```python
from build123d import *

# Parameters (mm, degrees)
SKETCH_1_R      = 1.5
SKETCH_1_R_2    = 7.9
SKETCH_1_R_3    = 1.25
SKETCH_1_W      = 6
SKETCH_1_H      = 10
SKETCH_1_W_2    = 10
SKETCH_1_H_2    = 6
EXTRUDE_1_DEPTH = 6


with BuildPart() as part:
    # Эскиз1 → Бобышка-Вытянуть1 (new body)
    with BuildSketch(Plane.XY):
        with BuildLine():
            Line((146.861398458, 191.532325026), (172.897783364, 191.532325026))
            ThreePointArc((172.897783364, 191.532325026), (177.076317747, 189.745999648), (178.804179186, 185.542952802))
            Line((178.804179186, 185.542952802), (178.804179186, -196.675834418))
            ThreePointArc((178.804179186, -196.675834418), (176.892140189, -200.429470569), (172.897783364, -201.767674974))
            Line((172.897783364, -201.767674974), (145.861398458, -201.767674974))
            ThreePointArc((145.861398458, -201.767674974), (142.269143233, -200.971291164), (139.350020692, -198.731369657))
            Line((139.350020692, -198.731369657), (137.054194639, -195.711716561))
            ThreePointArc((137.054194639, -195.711716561), (134.135072097, -193.471795054), (130.542816872, -192.675411244))
            Line((130.542816872, -192.675411244), (-129.747250144, -192.675411244))
            ThreePointArc((-129.747250144, -192.675411244), (-133.339505369, -193.471795054), (-136.258627911, -195.711716561))
            Line((-136.258627911, -195.711716561), (-138.554453964, -198.731369657))
            ThreePointArc((-138.554453964, -198.731369657), (-141.473576506, -200.971291164), (-145.06583173, -201.767674974))
            Line((-145.06583173, -201.767674974), (-172.102216636, -201.767674974))
            ThreePointArc((-172.102216636, -201.767674974), (-176.405497525, -200.043755719), (-178.195820814, -195.767674974))
            Line((-178.195820814, -195.767674974), (-178.195820814, 185.542952802))
            ThreePointArc((-178.195820814, 185.542952802), (-176.401714686, 189.812135315), (-172.102216636, 191.532325026))
            Line((-172.102216636, 191.532325026), (-146.06583173, 191.532325026))
            ThreePointArc((-146.06583173, 191.532325026), (-142.473576506, 192.328708836), (-139.554453964, 194.568630343))
            Line((-139.554453964, 194.568630343), (-136.258627911, 198.496442883))
            ThreePointArc((-136.258627911, 198.496442883), (-133.339449219, 200.73613298), (-129.747250144, 201.532325026))
            Line((-129.747250144, 201.532325026), (130.542816872, 201.532325026))
            ThreePointArc((130.542816872, 201.532325026), (134.135072097, 200.735941215), (137.054194639, 198.496019708))
            Line((137.054194639, 198.496019708), (140.350020692, 194.568207169))
            ThreePointArc((140.350020692, 194.568207169), (143.269199383, 192.328517071), (146.861398458, 191.532325026))
        make_face()
        with Locations((120.494179186, -138.767674974)):
            Circle(SKETCH_1_R, mode=Mode.SUBTRACT)
        with Locations((0.304179186, -138.767674974)):
            Circle(SKETCH_1_R, mode=Mode.SUBTRACT)
        with Locations((-119.885820814, -138.767674974)):
            Circle(SKETCH_1_R, mode=Mode.SUBTRACT)
        with Locations((-171.195820814, -116.737674974)):
            Circle(SKETCH_1_R, mode=Mode.SUBTRACT)
        with Locations((-171.195820814, 14.972325026)):
            Circle(SKETCH_1_R, mode=Mode.SUBTRACT)
        with Locations((171.804179186, 149.132325026)):
            Circle(SKETCH_1_R, mode=Mode.SUBTRACT)
        with Locations((126.444179186, 194.532325026)):
            Circle(SKETCH_1_R, mode=Mode.SUBTRACT)
        with Locations((-151.995820814, 178.532325026)):
            Circle(SKETCH_1_R_2, mode=Mode.SUBTRACT)
        with Locations((171.804179186, -116.737674974)):
            Circle(SKETCH_1_R, mode=Mode.SUBTRACT)
        with Locations((171.804179186, 14.972325026)):
            Circle(SKETCH_1_R, mode=Mode.SUBTRACT)
        with Locations((-171.195820814, 149.132325026)):
            Circle(SKETCH_1_R, mode=Mode.SUBTRACT)
        with Locations((-125.835820814, 194.532325026)):
            Circle(SKETCH_1_R, mode=Mode.SUBTRACT)
        with Locations((0.304179186, 194.54440539)):
            Circle(SKETCH_1_R, mode=Mode.SUBTRACT)
        with Locations((131.504179186, 178.532325026)):
            Circle(SKETCH_1_R_2, mode=Mode.SUBTRACT)
        with Locations((-139.995820814, 178.532325026)):
            Circle(SKETCH_1_R_3, mode=Mode.SUBTRACT)
        with Locations((-163.995820814, 178.532325026)):
            Circle(SKETCH_1_R_3, mode=Mode.SUBTRACT)
        with Locations((119.504179186, 178.532325026)):
            Circle(SKETCH_1_R_3, mode=Mode.SUBTRACT)
        with Locations((143.504179186, 178.532325026)):
            Circle(SKETCH_1_R_3, mode=Mode.SUBTRACT)
        with Locations((-171.195820814, 39.972325026)):
            Rectangle(SKETCH_1_W, SKETCH_1_H, mode=Mode.SUBTRACT)
        with Locations((171.804179186, 39.972325026)):
            Rectangle(SKETCH_1_W, SKETCH_1_H, mode=Mode.SUBTRACT)
        Polygon((174.804179186, 179.132325026), (174.804179186, 169.359038573), (174.804179186, 169.132325026), (168.804179186, 169.132325026), (168.804179186, 179.132325026), align=None, mode=Mode.SUBTRACT)
        Polygon((96.444179186, 197.532325026), (106.41988356, 197.532325026), (106.444179186, 197.514906712), (106.444179186, 191.332537312), (106.419882773, 191.532325026), (96.444179186, 191.532325026), align=None, mode=Mode.SUBTRACT)
        with Locations((26.094179186, -138.767674974)):
            Rectangle(SKETCH_1_W_2, SKETCH_1_H_2, mode=Mode.SUBTRACT)
        with Locations((-25.485820814, -138.767674974)):
            Rectangle(SKETCH_1_W_2, SKETCH_1_H_2, mode=Mode.SUBTRACT)
        with Locations((-171.195820814, 174.132325026)):
            Rectangle(SKETCH_1_W, SKETCH_1_H, mode=Mode.SUBTRACT)
        with Locations((94.094179186, -138.767674974)):
            Rectangle(SKETCH_1_W_2, SKETCH_1_H_2, mode=Mode.SUBTRACT)
        with Locations((146.894179186, -138.767674974)):
            Rectangle(SKETCH_1_W_2, SKETCH_1_H_2, mode=Mode.SUBTRACT)
        Polygon((-19.68524425, 191.532325026), (-29.685244433, 191.532325026), (-29.686393667, 197.532325026), (-19.686393484, 197.532325026), align=None, mode=Mode.SUBTRACT)
        with Locations((-171.195820814, 124.132325026)):
            Rectangle(SKETCH_1_W, SKETCH_1_H, mode=Mode.SUBTRACT)
        with Locations((-146.285820814, -138.767674974)):
            Rectangle(SKETCH_1_W_2, SKETCH_1_H_2, mode=Mode.SUBTRACT)
        with Locations((25.294179186, 194.532325026)):
            Rectangle(SKETCH_1_W_2, SKETCH_1_H_2, mode=Mode.SUBTRACT)
        with Locations((-171.195820814, -10.027674974)):
            Rectangle(SKETCH_1_W, SKETCH_1_H, mode=Mode.SUBTRACT)
        with Locations((-171.195820814, -91.757674974)):
            Rectangle(SKETCH_1_W, SKETCH_1_H, mode=Mode.SUBTRACT)
        with Locations((-171.195820814, -141.747674974)):
            Rectangle(SKETCH_1_W, SKETCH_1_H, mode=Mode.SUBTRACT)
        with Locations((-93.485820814, -138.767674974)):
            Rectangle(SKETCH_1_W_2, SKETCH_1_H_2, mode=Mode.SUBTRACT)
        with Locations((171.804179186, -10.027674974)):
            Rectangle(SKETCH_1_W, SKETCH_1_H, mode=Mode.SUBTRACT)
        with Locations((171.804179186, -91.757674974)):
            Rectangle(SKETCH_1_W, SKETCH_1_H, mode=Mode.SUBTRACT)
        with Locations((171.804179186, -141.747674974)):
            Rectangle(SKETCH_1_W, SKETCH_1_H, mode=Mode.SUBTRACT)
        with Locations((171.804179186, 124.132325026)):
            Rectangle(SKETCH_1_W, SKETCH_1_H, mode=Mode.SUBTRACT)
        Polygon((-95.835245647, 191.532325026), (-105.83524583, 191.532325026), (-105.836395064, 197.532325026), (-95.836394881, 197.532325026), align=None, mode=Mode.SUBTRACT)
        with BuildLine():
            Line((-128.195820814, -73.467674974), (-128.195820814, 51.532325026))
            ThreePointArc((-128.195820814, 51.532325026), (-98.906498933, 122.243003144), (-28.195820814, 151.532325026))
            Line((-28.195820814, 151.532325026), (81.804179186, 151.532325026))
            ThreePointArc((81.804179186, 151.532325026), (88.875246998, 148.603392838), (91.804179186, 141.532325026))
            Line((91.804179186, 141.532325026), (91.804179186, -73.467674974))
            ThreePointArc((91.804179186, -73.467674974), (88.875246998, -80.538742786), (81.804179186, -83.467674974))
            Line((81.804179186, -83.467674974), (-118.195820814, -83.467674974))
            ThreePointArc((-118.195820814, -83.467674974), (-125.266888626, -80.538742786), (-128.195820814, -73.467674974))
        make_face(mode=Mode.SUBTRACT)
    extrude(amount=EXTRUDE_1_DEPTH)


solid = part.part
```
Design review of the part built by this model. Coordinates are the model's own, in mm. A direction names the side the tool comes from. Give positions to 0.01 mm unless a question says otherwise; leave off trailing zeros. Write each loop counter-clockwise with the first axis right and the second up, starting at its lowest first coordinate (ties: lowest second). Pieces come first, ordered by that corner, then holes.
(1) Add section C-C (z = 2.85). Give the number of separate pieces and of enclosed holes in the cut face, and give its area (3 significant figures).
Checked values:
separate pieces: 1
enclosed holes: 41
area: 89,300 mm2
(2) Clearance check with a flat-ended pin moving along its axis: pin 1 Ø3 at (x, z) = (24, 3.5) entering from -Y. State where the tip first meets the part, or that it passes through.
Checked values:
pin 1: stops at y = -192.68
(3) Mouldability with a two-part tool opening along Y and no side actions: class faces 1 (the face through (88.8, 148.68, 2.96)), 2 (the face through (3, -87, 0)) as +Y half, -Y half, draft (parallel to the pull), parting line (faces both ways), or undercut.
Checked values:
face 1: undercut
face 2: draft
(4) Add section A-A (x = 54). Give the boundary of the cut face in (y, z), and give its area (3 significant figures).
Checked values:
outline: (-192.68, 0) - (-83.47, 0) - (-83.47, 6) - (-192.68, 6) - close; (151.53, 0) - (201.53, 0) - (201.53, 6) - (151.53, 6) - close
area: 955 mm2
(5) Add section B-B (y = -64). Give the boundary of the cut face in (x, z), and give its area (3 significant figures).
Checked values:
outline: (-178.2, 0) - (-128.2, 0) - (-128.2, 6) - (-178.2, 6) - close; (91.8, 0) - (178.8, 0) - (178.8, 6) - (91.8, 6) - close
area: 822 mm2
(6) Wall thickness on line 1 along Y through (x, z) = (-22.5, 1.8); line 2 along X through (y, z) = (184, 0.45); line 3 along Y through (x, z) = (-31, 3.2): over which ranges is each line inside the solid? List them lowest first.
Checked values:
line 1: y = -192.68 to -141.77, -135.77 to -83.47, 151.53 to 191.53, 197.53 to 201.53
line 2: x = -178.2 to -157.7, -146.29 to 125.8, 137.21 to 178.8
line 3: y = -192.68 to -83.47, 151.49 to 201.53
(7) Tool access review of faces 3 (the face through (-99.68, 121.46, 2.96)), 4 (the face through (3, -87, 6)): name each direction out of +Z, -Z, +X, -X, +Y, -Y from which nothing blocks a thin tool from reaching the whole face with its end or side.
Checked values:
face 3: +Z, -Z
face 4: +Z, +X, -X, +Y, -Y
